from build123d import *

# Parameters (mm, degrees)
SKETCH1_W                      = 38
SKETCH1_H                      = 30
BASE_FLANGE1_DEPTH             = 0.8
EDGE_FLANGE1_STRIP_W           = 4.8
EDGE_FLANGE1_STRIP_H           = 0.8
EDGE_FLANGE1_STRIP_CUT_DEPTH   = 30
EDGE_FLANGE1_STRIP_2_W         = 4.8
EDGE_FLANGE1_STRIP_2_H         = 0.8
EDGE_FLANGE1_STRIP_CUT_2_DEPTH = 30
EDGE_FLANGE1_DEPTH             = 30
EDGE_FLANGE1_BEND_DEPTH        = 30
EDGE_FLANGE2_STRIP_W           = 4.8
EDGE_FLANGE2_STRIP_H           = 0.8
EDGE_FLANGE2_STRIP_CUT_DEPTH   = 30
EDGE_FLANGE2_STRIP_2_W         = 4.8
EDGE_FLANGE2_STRIP_2_H         = 0.8
EDGE_FLANGE2_STRIP_CUT_2_DEPTH = 30
EDGE_FLANGE2_DEPTH             = 30
EDGE_FLANGE2_BEND_DEPTH        = 30
SKETCH15_R                     = 2
CUT_EXTRUDE1_DEPTH             = 10


# Sheet-metal steps are written as plain solids
with BuildPart() as part:
    # Sketch1 → Base-Flange1 (new body)
    with BuildSketch(Plane(origin=(0, 0, 0), x_dir=(1, 0, 0), z_dir=(0, 1, 0))):
        Rectangle(SKETCH1_W, SKETCH1_H)
    extrude(amount=-BASE_FLANGE1_DEPTH)

    # Edge-Flange1 strip (across the edge) → Edge-Flange1 strip cut (cut)
    with BuildSketch(Plane(origin=(-19, -0.8, 15), x_dir=(1, 0, 0), z_dir=(0, 0, -1))):
        with Locations((-0.8, -0.4)):
            Rectangle(EDGE_FLANGE1_STRIP_W, EDGE_FLANGE1_STRIP_H)
    extrude(amount=EDGE_FLANGE1_STRIP_CUT_DEPTH, mode=Mode.SUBTRACT)

    # Edge-Flange1 strip 2 (across the edge) → Edge-Flange1 strip cut 2 (cut)
    with BuildSketch(Plane(origin=(19, -0.8, -15), x_dir=(-1, 0, 0), z_dir=(0, 0, 1))):
        with Locations((-0.8, -0.4)):
            Rectangle(EDGE_FLANGE1_STRIP_2_W, EDGE_FLANGE1_STRIP_2_H)
    extrude(amount=EDGE_FLANGE1_STRIP_CUT_2_DEPTH, mode=Mode.SUBTRACT)

    # Edge-Flange1 section (across the edge) → Edge-Flange1 (add)
    with BuildSketch(Plane(origin=(-19, -0.8, 15), x_dir=(1, 0, 0), z_dir=(0, 0, -1))):
        with BuildLine():
            Line((0, 0.8), (0, 38.2))
            Line((0, 38.2), (0.8, 38.2))
            Line((0.8, 38.2), (0.8, 0.8))
            ThreePointArc((0.8, 0.8), (1.034314575, 0.234314575), (1.6, 0))
            Line((1.6, 0), (1.6, -0.8))
            ThreePointArc((1.6, -0.8), (0.46862915, -0.33137085), (0, 0.8))
        make_face()
    extrude(amount=EDGE_FLANGE1_DEPTH)

    # Edge-Flange1 section 2 (across the edge) → Edge-Flange1 bend (add)
    with BuildSketch(Plane(origin=(19, -0.8, -15), x_dir=(-1, 0, 0), z_dir=(0, 0, 1))):
        with BuildLine():
            Line((0, 0.8), (0, 38.2))
            Line((0, 38.2), (0.8, 38.2))
            Line((0.8, 38.2), (0.8, 0.8))
            ThreePointArc((0.8, 0.8), (1.034314575, 0.234314575), (1.6, 0))
            Line((1.6, 0), (1.6, -0.8))
            ThreePointArc((1.6, -0.8), (0.46862915, -0.33137085), (0, 0.8))
        make_face()
    extrude(amount=EDGE_FLANGE1_BEND_DEPTH)

    # Edge-Flange2 strip (across the edge) → Edge-Flange2 strip cut (cut)
    with BuildSketch(Plane(origin=(-19, -39, -15), x_dir=(0, 1, 0), z_dir=(0, 0, 1))):
        with Locations((-0.8, -0.4)):
            Rectangle(EDGE_FLANGE2_STRIP_W, EDGE_FLANGE2_STRIP_H)
    extrude(amount=EDGE_FLANGE2_STRIP_CUT_DEPTH, mode=Mode.SUBTRACT)

    # Edge-Flange2 strip 2 (across the edge) → Edge-Flange2 strip cut 2 (cut)
    with BuildSketch(Plane(origin=(19, -39, 15), x_dir=(0, 1, 0), z_dir=(0, 0, -1))):
        with Locations((-0.8, -0.4)):
            Rectangle(EDGE_FLANGE2_STRIP_2_W, EDGE_FLANGE2_STRIP_2_H)
    extrude(amount=EDGE_FLANGE2_STRIP_CUT_2_DEPTH, mode=Mode.SUBTRACT)

    # Edge-Flange2 section (across the edge) → Edge-Flange2 (add)
    with BuildSketch(Plane(origin=(-19, -39, -15), x_dir=(0, 1, 0), z_dir=(0, 0, 1))):
        with BuildLine():
            Line((0, 0.8), (0, 9.2))
            Line((0, 9.2), (0.8, 9.2))
            Line((0.8, 9.2), (0.8, 0.8))
            ThreePointArc((0.8, 0.8), (1.034314575, 0.234314575), (1.6, 0))
            Line((1.6, 0), (1.6, -0.8))
            ThreePointArc((1.6, -0.8), (0.46862915, -0.33137085), (0, 0.8))
        make_face()
    extrude(amount=EDGE_FLANGE2_DEPTH)

    # Edge-Flange2 section 2 (across the edge) → Edge-Flange2 bend (add)
    with BuildSketch(Plane(origin=(19, -39, 15), x_dir=(0, 1, 0), z_dir=(0, 0, -1))):
        with BuildLine():
            Line((0, 0.8), (0, 9.2))
            Line((0, 9.2), (0.8, 9.2))
            Line((0.8, 9.2), (0.8, 0.8))
            ThreePointArc((0.8, 0.8), (1.034314575, 0.234314575), (1.6, 0))
            Line((1.6, 0), (1.6, -0.8))
            ThreePointArc((1.6, -0.8), (0.46862915, -0.33137085), (0, 0.8))
        make_face()
    extrude(amount=EDGE_FLANGE2_BEND_DEPTH)

    # Sketch15 → Cut-Extrude1 (cut)
    with BuildSketch(Plane(origin=(0, -38.2, 0), x_dir=(1, 0, 0), z_dir=(0, 1, 0))):
        with Locations(Location((-23.7, 0, 0), (0, 0, 270))):
            Circle(SKETCH15_R)
        with Locations(Location((23.7, 0, 0), (0, 0, 270))):
            Circle(SKETCH15_R)
    extrude(amount=-CUT_EXTRUDE1_DEPTH, mode=Mode.SUBTRACT)


solid = part.part
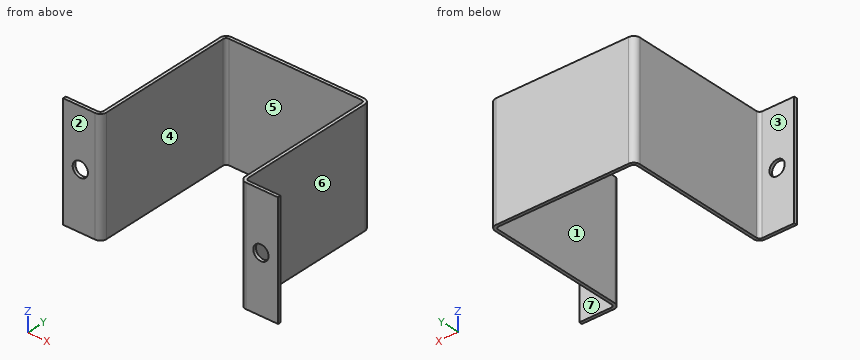
Could you check a few things on this model? Use its own coordinates, in mm. Face numbers are marked on the shaded views. A direction names the side the tool comes from. Give positions to 0.01 mm unless a question says otherwise; leave off trailing zeros. Order: outer loops, then holes, each group sorted by start corner. A loop starts at its lowest first (then second) coordinate and runs counter-clockwise, first axis right, second up. Notation, with made-up numbers: (52.25, 28) - (68.25, 28) arc R14 cw to (68.25, 45) - close; hole circle Ø2 at (72, 50.25). An arc over 180 degrees is marked (long way). Return JSON: item names as keys, results as strings. Group by question number.
Q1. Which directions (+Z, -Z, +X, -X, +Y, -Y) give clear straight access to the entire face, cutting with the end or side of a thin tool? Please do the marked faces 1, 2 and 3.
Q2. Suppose I cut it at D-D, the plane z = -3. Please give me the cut outline in (x, y).
Q3. Suppose I cut it at C-C, the plane x = -23.7. Please give me the cut outline in (y, z), and give its area (3 significant figures).
Q4. Please list where these lines run through material, in increasing order: line 1 along X through (y, z) = (-19.5, 7.5); line 2 along X through (y, z) = (-38.6, 0); line 3 along X through (y, z) = (-38.65, 0). Write a range as [from, to].
Q5. Thinking about a two-plate mould opening in X: for the marked faces 4, 5, 6 and 7, which applies, pulls with the +X half, pulls with the -X half, needs draft (parallel to the pull), parting line crosses it, or undercut?
Q6. Suppose I cut it at B-B, the plane y = -23. Please give me the cut outline in (x, z), and give its area (3 significant figures).
Q7. Will these pins go through, and if not, where does the flat tip stop? pin 1 Ø15 at (y, z) = (-14.5, 0.5) entering from -X; pin 2 Ø2 at (y, z) = (-13.5, -1.5) entering from +X; pin 3 Ø4.5 at (x, z) = (23.7, 0) entering from +Y.
Q8. Suppose I cut it at A-A, the plane z = 0. Please give me the cut outline in (x, y), and give its area (3 significant figures).
Resolved:
{
 "1": {"face 1": "+Z, -Z, -Y", "face 2": "+Z, -Z, +X, -X, -Y", "face 3": "+Z, -Z, -X, +Y"},
 "2": {"outline": "(-28.2, -39) - (-19.8, -39) arc R1.6 ccw to (-18.2, -37.4) - (-18.2, -1.6) arc R0.8 cw to (-17.4, -0.8) - (17.4, -0.8) arc R0.8 cw to (18.2, -1.6) - (18.2, -37.4) arc R1.6 ccw to (19.8, -39) - (28.2, -39) - (28.2, -38.2) - (19.8, -38.2) arc R0.8 cw to (19, -37.4) - (19, -1.6) arc R1.6 ccw to (17.4, 0) - (-17.4, 0) arc R1.6 ccw to (-19, -1.6) - (-19, -37.4) arc R0.8 cw to (-19.8, -38.2) - (-28.2, -38.2) - close"},
 "3": {"outline": "(-39, -15) - (-38.2, -15) - (-38.2, -2) - (-39, -2) - close; (-39, 2) - (-38.2, 2) - (-38.2, 15) - (-39, 15) - close", "area": "20.8 mm2"},
 "4": {"line 1": "x = [-19, -18.2], [18.2, 19]", "line 2": "x = [-28.2, -25.7], [-21.7, -18.74], [18.74, 21.7], [25.7, 28.2]", "line 3": "x = [-28.2, -25.7], [-21.7, -18.8], [18.8, 21.7], [25.7, 28.2]"},
 "5": {"face 4": "undercut", "face 5": "undercut", "face 6": "pulls with the +X half", "face 7": "needs draft"},
 "6": {"outline": "(-19, -15) - (-18.2, -15) - (-18.2, 15) - (-19, 15) - close; (18.2, -15) - (19, -15) - (19, 15) - (18.2, 15) - close", "area": "48.0 mm2"},
 "7": {"pin 1": "stops at x = -19", "pin 2": "stops at x = 19", "pin 3": "stops at y = -38.2"},
 "8": {"outline": "(-28.2, -39) - (-25.7, -39) - (-25.7, -38.2) - (-28.2, -38.2) - close; (-21.7, -39) - (-19.8, -39) arc R1.6 ccw to (-18.2, -37.4) - (-18.2, -1.6) arc R0.8 cw to (-17.4, -0.8) - (17.4, -0.8) arc R0.8 cw to (18.2, -1.6) - (18.2, -37.4) arc R1.6 ccw to (19.8, -39) - (21.7, -39) - (21.7, -38.2) - (19.8, -38.2) arc R0.8 cw to (19, -37.4) - (19, -1.6) arc R1.6 ccw to (17.4, 0) - (-17.4, 0) arc R1.6 ccw to (-19, -1.6) - (-19, -37.4) arc R0.8 cw to (-19.8, -38.2) - (-21.7, -38.2) - close; (25.7, -39) - (28.2, -39) - (28.2, -38.2) - (25.7, -38.2) - close", "area": "98.2 mm2"}
}
